from build123d import *

# Parameters (mm, degrees)
SKETCH003_W   = 39
SKETCH003_H   = 21.5
SKETCH003_W_2 = 30
SKETCH003_H_2 = 5.5
PAD003_DEPTH  = 10
SKETCH004_W   = 36
SKETCH004_H   = 20.5
POCKET_DEPTH  = 10
CHAMFER_SIZE2 = 7
CHAMFER_SIZE  = 1.5


with BuildPart() as part:
    # Sketch003 → Pad003 (new body)
    with BuildSketch(Plane.XY.offset(13)):
        with Locations((17.5, -76.25)):
            Rectangle(SKETCH003_W, SKETCH003_H)
        with Locations((17.5, -80.5)):
            Rectangle(SKETCH003_W_2, SKETCH003_H_2, mode=Mode.SUBTRACT)
    extrude(amount=PAD003_DEPTH)

    # Sketch004 → Pocket (cut)
    with BuildSketch(Plane.XY.offset(15.5)):
        with Locations((17, -75.75)):
            Rectangle(SKETCH004_W, SKETCH004_H)
    extrude(amount=-POCKET_DEPTH, mode=Mode.SUBTRACT)

    # Chamfer
    chamfer_edges = [part.edges().sort_by_distance(p)[0] for p in [
        (17.5, -77.75, 23),
        (17.5, -83.25, 23),
    ]]
    chamfer_side = part.faces().sort_by_distance((17.5, -75.208797, 23))[0]
    chamfer(chamfer_edges, length=CHAMFER_SIZE, length2=CHAMFER_SIZE2, reference=chamfer_side)


solid = part.part
Design review of the part built by this model. Coordinates are the model's own, in mm. A direction names the side the tool comes from. Coordinates: 2 decimals unless noted, no trailing zeros. Loops run counter-clockwise (first coordinate to the right, second up) from the corner with the lowest first, then second, coordinate; pieces in that order, holes last. Notation, with made-up numbers: (24, 82) -> (39, 82) arc R28 cw to (39, 105) -> close; hole circle Ø10 at (33, 64). An arc over 180 degrees is marked (long way). Use a Markdown table: item, result. Add a question column.
Item 1: We need section C-C, the plane y = -77. Write out the cut boundary in (x, z), and give its area (3 significant figures).
Item 2: Wall thickness on L1, parallel to X at y = -73, z = 13.75; L2, parallel to X at y = -81.5, z = 16.25; L3, parallel to Z at x = 24.5, y = -73.75: over which ranges is each line inside the solid? List them lowest first. Write a range as from..to.
Item 3: The part is to be moulded in two halves that separate along X. For faces 1 (the flat face through (2.5, -81, 19)), 2 (the flat face through (17.4, -86.6, 13)), 3 (the flat face through (37, -76, 18)), 4 (the flat face through (35, -76, 14)), say which applies: +X half, -X half, draft (parallel to the pull), parting line (faces both ways), or undercut.
Item 4: We need section D-D, the plane z = 18. Write out the cut boundary in (x, y).
Item 5: We need section B-B, the plane x = 24. Write out the cut boundary in (y, z).
Item 6: We need section A-A, the plane y = -80. Write out the cut boundary in (x, z), and give its area (3 significant figures).
Item 7: Clearance check with flat-ended pins moving along their axes: P1, Ø5, axis at x = 25, y = -74.5, coming from the -Z side; P2, Ø1.2, axis at x = 18, z = 14, coming from the +Y side. State where each tip first meets the part, or that it passes through.
Item 8: Machinability: for faces 5 (the flat face through (17.3, -84, 19.5)), 6 (the flat face through (-1, -76, 14)), 7 (the flat face through (17, -65.5, 19)), which of the approach directions +Z, -Z, +X, -X, +Y, -Y give a long, thin tool a straight path to every point of the face, cutting with its end or side? Answer none if there is none.
Numbers:
| question | item | result |
|---|---|---|
| 1 | outline | (-2, 13) -> (-1, 13) -> (-1, 15.5) -> (35, 15.5) -> (35, 13) -> (37, 13) -> (37, 23) -> (32.5, 23) -> (32.5, 19.5) -> (2.5, 19.5) -> (2.5, 23) -> (-2, 23) -> close |
| 1 | area | 195 mm^2 |
| 2 | L1 | x = -2..-1, 35..37 |
| 2 | L2 | x = -2..2.5, 32.5..37 |
| 2 | L3 | z = 15.5..23 |
| 3 | face 1 | undercut |
| 3 | face 2 | draft |
| 3 | face 3 | +X half |
| 3 | face 4 | undercut |
| 4 | outline | (-2, -87) -> (37, -87) -> (37, -65.5) -> (-2, -65.5) -> close; hole (2.5, -83.68) -> (32.5, -83.68) -> (32.5, -77.32) -> (2.5, -77.32) -> close |
| 5 | outline | (-87, 13) -> (-86, 13) -> (-86, 15.5) -> (-83.25, 15.5) -> (-83.25, 16) -> (-84.75, 23) -> (-87, 23) -> close; (-77.75, 15.5) -> (-65.5, 15.5) -> (-65.5, 23) -> (-76.25, 23) -> (-77.75, 16) -> close |
| 6 | outline | (-2, 13) -> (-1, 13) -> (-1, 15.5) -> (2.5, 15.5) -> (2.5, 23) -> (-2, 23) -> close; (32.5, 15.5) -> (35, 15.5) -> (35, 13) -> (37, 13) -> (37, 23) -> (32.5, 23) -> close |
| 6 | area | 75.0 mm^2 |
| 7 | P1 | stops at z = 15.5 |
| 7 | P2 | stops at y = -86 |
| 8 | face 5 | +Z |
| 8 | face 6 | -Z, +Y |
| 8 | face 7 | +Z, -Z, +X, -X, +Y |
